CAD build for the part. Positions are in the model's coordinates, mm. A direction names the side the tool comes from. Give positions to 0.01 mm unless a question says otherwise; leave off trailing zeros. Loops run counter-clockwise (first coordinate to the right, second up) from the corner with the lowest first, then second, coordinate; pieces in that order, holes last.
Item 1: Saw through at D-D on x = -13. Give the cut face in (y, z), plus the area to 3 significant figures.
Item 2: Saw through at C-C on y = -30. Give the cut face in (x, z).
Item 3: Saw through at B-B on x = -26.5. Give the cut face in (y, z), plus the area to 3 significant figures.
Item 4: Which spindle directions (+Z, -Z, +X, -X, +Y, -Y) get a long thin tool onto all of the face, cutting with end or side? Do faces 5 (the flat face through (-26, 48.049, -1)), 6 (the cylindrical face through (-36.178, 51.409, -1.479)), 7 (the cylindrical face through (-48.17, -41.82, 9.96)), 8 (the flat face through (-25, 7, 17)), 9 (the cylindrical face through (-15.237, 51.264, -1.479)). Say none if no direction does.
Item 5: Saw through at A-A on z = 14.5. Give the cut face in (x, y).
Item 6: Probe probe 1 along Y at (x, z) = (-26.5, 12.25); probe 2 along X at (y, z) = (-9.5, 9.25); probe 3 along Z at (x, y) = (-7, 21). List the from-to ranges inside material, lowest first.
Item 7: Mould opens along Y. For faces 1 (the flat face through (-54, -39.281, 10)), 2 (the flat face through (-58, 2, 0)), 3 (the flat face through (-26, 54.624, -1)), 4 (the flat face through (6.981, 6, 8)) say: released by +Y, released by -Y, zero draft, split by the parting line, or undercut.
Item 8: Drop flat-ended pins along their axis: P1, Ø2.5, axis at x = -29, z = -1.5, coming from the -Y side; P2, Ø7, axis at x = -0.5, y = 51, coming from the -Z side; P3, Ø2.5, axis at x = -23.5, z = -1.5, coming from the +Y side; P4, Ø2.5, axis at x = -53, z = 9.5, coming from the -Y side. Give the stop position or say it passes through.
from build123d import *

# Parameters (mm, degrees)
SKETCH1_W           = 80
SKETCH1_H           = 100
BOSS_EXTRUDE1_DEPTH = 20
SKETCH2_W           = 64
SKETCH2_H           = 80
CUT_EXTRUDE1_DEPTH  = 17
BOSS_EXTRUDE2_DEPTH = 3
SKETCH5_R           = 3.199851011
CUT_EXTRUDE2_DEPTH  = 2.7
CUT_EXTRUDE3_DEPTH  = 5


with BuildPart() as part:
    # Sketch1 → Boss-Extrude1 (new body)
    with BuildSketch(Plane.XY):
        with Locations((-25.342231874, 5.71880103)):
            Rectangle(SKETCH1_W, SKETCH1_H)
    extrude(amount=BOSS_EXTRUDE1_DEPTH)

    # Sketch2 → Cut-Extrude1 (cut)
    with BuildSketch(Plane(origin=(0, 0, 0), x_dir=(-1, 0, 0), z_dir=(0, 0, -1))):
        with Locations((25.018703927, 6.11109777)):
            Rectangle(SKETCH2_W, SKETCH2_H)
    extrude(amount=-CUT_EXTRUDE1_DEPTH, mode=Mode.SUBTRACT)

    # Sketch3 → Boss-Extrude2 (add)
    with BuildSketch(Plane(origin=(0, 0, 0), x_dir=(-1, 0, 0), z_dir=(0, 0, -1))):
        with BuildLine():
            Line((18.523780304, 54.623908994), (32.891231828, 54.623908994))
            ThreePointArc((32.891231828, 54.623908994), (36.178699549, 51.336441272), (32.891231828, 48.048973551))
            Line((32.891231828, 48.048973551), (18.523780304, 48.048973551))
            ThreePointArc((18.523780304, 48.048973551), (15.236312582, 51.336441272), (18.523780304, 54.623908994))
        make_face()
    extrude(amount=BOSS_EXTRUDE2_DEPTH)

    # Sketch5 → Cut-Extrude2 (cut)
    with BuildSketch(Plane(origin=(0, 0, 0), x_dir=(-1, 0, 0), z_dir=(0, 0, -1))):
        with Locations((-0.897871535, 51.161432221)):
            Circle(SKETCH5_R)
    extrude(amount=-CUT_EXTRUDE2_DEPTH, mode=Mode.SUBTRACT)

    # Sketch8 → Cut-Extrude3 (cut)
    with BuildSketch(Plane.XZ.offset(44.28119897)):
        with BuildLine():
            Line((-58.0956261, 11.534398485), (-49.77573211, 11.534398485))
            ThreePointArc((-49.77573211, 11.534398485), (-48.168479863, 9.927146237), (-49.77573211, 8.319893989))
            Line((-49.77573211, 8.319893989), (-58.0956261, 8.319893989))
            ThreePointArc((-58.0956261, 8.319893989), (-59.702878348, 9.927146237), (-58.0956261, 11.534398485))
        make_face()
    extrude(amount=-CUT_EXTRUDE3_DEPTH, mode=Mode.SUBTRACT)


solid = part.part
Results below:
1. outline: (-44.28, 0) - (-33.89, 0) - (-33.89, 17) - (46.11, 17) - (46.11, 0) - (55.72, 0) - (55.72, 20) - (-44.28, 20) - close
1. area: 640 mm2
2. outline: (-65.34, 0) - (-57.02, 0) - (-57.02, 17) - (6.98, 17) - (6.98, 0) - (14.66, 0) - (14.66, 20) - (-65.34, 20) - close
3. outline: (-44.28, 0) - (-33.89, 0) - (-33.89, 17) - (46.11, 17) - (46.11, 0) - (48.05, 0) - (48.05, -3) - (54.62, -3) - (54.62, 0) - (55.72, 0) - (55.72, 20) - (-44.28, 20) - close
3. area: 660 mm2
4. face 5: -Z, +X, -X, -Y
4. face 6: -Z, -X
4. face 7: -Y
4. face 8: -Z
4. face 9: -Z, +X
5. outline: (-65.34, -44.28) - (14.66, -44.28) - (14.66, 55.72) - (-65.34, 55.72) - close; hole (-57.02, -33.89) - (6.98, -33.89) - (6.98, 46.11) - (-57.02, 46.11) - close
6. probe 1: y = -44.28 to -33.89, 46.11 to 55.72
6. probe 2: x = -65.34 to -57.02, 6.98 to 14.66
6. probe 3: z = 17 to 20
7. face 1: released by -Y
7. face 2: zero draft
7. face 3: released by +Y
7. face 4: undercut
8. P1: stops at y = 48.05
8. P2: stops at z = 0
8. P3: stops at y = 54.62
8. P4: stops at y = -44.28
